Part model, mm, in its own coordinate system. Face numbers are marked on the shaded views. A direction names the side the tool comes from. Coordinates: 2 decimals unless noted, no trailing zeros. Loops run counter-clockwise (first coordinate to the right, second up) from the corner with the lowest first, then second, coordinate; pieces in that order, holes last.
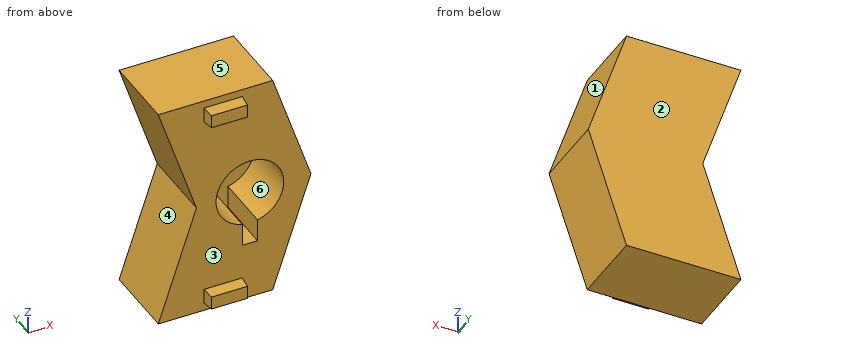
```python
from build123d import *

# Parameters (mm, degrees)
BOSS_EXTRUDE1_DEPTH       = 12.7
SKETCH2_R                 = 5.635000033
HAPTIC_MOTOR_CUTOUT_DEPTH = 9.557999934
SKETCH3_W                 = 2.54
SKETCH3_H                 = 3.81
HAPTIC_WIRE_CUTOUT_DEPTH  = 9.557999934
SKETCH4_W                 = 6.35
SKETCH4_H                 = 2.54
PINS_DEPTH                = 2.032
PINS_TAPER                = 5


with BuildPart() as part:
    # Sketch1 → Boss-Extrude1 (new body)
    with BuildSketch(Plane(origin=(0, 0, 0), x_dir=(1, 0, 0), z_dir=(0, 1, 0))):
        Polygon((0, 0), (19.05, 0), (25.4, 19.05), (19.05, 38.1), (0, 38.1), (6.35, 19.05), align=None)
    extrude(amount=BOSS_EXTRUDE1_DEPTH)

    # Sketch2 → Haptic Motor Cutout (cut)
    with BuildSketch(Plane.XZ):
        with Locations((15.24, -19.05)):
            Circle(SKETCH2_R)
    extrude(amount=-HAPTIC_MOTOR_CUTOUT_DEPTH, mode=Mode.SUBTRACT)

    # Sketch3 → Haptic Wire Cutout (cut)
    with BuildSketch(Plane.XZ):
        with Locations((15.24, -26.445020526)):
            Rectangle(SKETCH3_W, SKETCH3_H)
    extrude(amount=-HAPTIC_WIRE_CUTOUT_DEPTH, mode=Mode.SUBTRACT)

    # Sketch4 → Pins (add)
    with BuildSketch(Plane.XZ):
        with Locations((10.795, -35.56)):
            Rectangle(SKETCH4_W, SKETCH4_H)
    pins = extrude(amount=PINS_DEPTH, taper=PINS_TAPER)

    # Mirror1: Pins across plane
    add(pins.mirror(Plane(origin=(0, 0, -19.05), x_dir=(1, 0, 0), z_dir=(0, 0, -1))))


solid = part.part
```
Q1. Probe line 1 (X direction, y = 6.25, z = -19.05) (3 decimals); line 2 (Z direction, x = 15.24, y = 5) (3 decimals); line 3 (Y direction, x = 17, z = -9.5). List the from-to ranges inside material, lowest first.
Q2. Saw through at B-B (y = 7). List the corners of the cut face in (x, z) (3 decimals).
Q3. Mould opens along Z. For the marked faces 1, 2 and 3 say: released by +Z, released by -Z, zero draft, split by the parting line, or undercut.
Q4. Saw through at A-A (x = 3.5). List the corners of the cut face in (y, z), plus the area to 3 significant figures.
Q5. Saw through at D-D (z = -19.5). List the corners of the cut face in (x, y), plus the area to 3 significant figures.
Q6. Saw through at C-C (x = 15.24). List the corners of the cut face in (y, z) (3 decimals), plus the area to 3 significant figures.
Q7. Tool access for the marked faces 4, 5 and 6: list every direction of +Z, -Z, +X, -X, +Y, -Y with a clear straight run to the whole face (end or side of a thin tool).
Q8. Drop flat-ended pins along their axis: P1, Ø3, axis at y = 4, z = -26.5, coming from the -X side; P2, Ø12.5, axis at x = 17, z = -14.5, coming from the -Y side; P3, Ø3, axis at y = 8, z = -18.5, coming from the -X side. Give the stop position or say it passes through.
Checked values:
1. line 1: x = 6.35 to 9.605, 20.875 to 25.4
1. line 2: z = -38.1 to -28.35, -13.415 to 0
1. line 3: y = 0 to 12.7
2. outline: (0, -38.1) - (19.05, -38.1) - (25.4, -19.05) - (19.05, 0) - (0, 0) - (6.35, -19.05) - close; hole (13.97, -28.35) - (16.51, -28.35) - (16.51, -24.54) arc R5.635 ccw (long way) to (13.97, -24.54) - close
3. face 1: released by +Z
3. face 2: zero draft
3. face 3: undercut
4. outline: (0, -38.1) - (12.7, -38.1) - (12.7, -27.6) - (0, -27.6) - close; (0, -10.5) - (12.7, -10.5) - (12.7, 0) - (0, 0) - close
4. area: 267 mm2
5. outline: (6.2, 0) - (9.62, 0) - (9.62, 9.56) - (20.86, 9.56) - (20.86, 0) - (25.25, 0) - (25.25, 12.7) - (6.2, 12.7) - close
5. area: 135 mm2
6. outline: (0, -38.1) - (12.7, -38.1) - (12.7, 0) - (0, 0) - (0, -13.415) - (9.558, -13.415) - (9.558, -28.35) - (0, -28.35) - close
6. area: 341 mm2
7. face 4: -X, +Y, -Y
7. face 5: +Z, +X, -X, +Y, -Y
7. face 6: -Y
8. P1: stops at x = 3.37
8. P2: stops at y = 0
8. P3: stops at x = 5.67
